```python
from build123d import *

# Parameters (mm, degrees)
F1_DEPTH = 101.6
F2_DEPTH = 12.7
F3_DEPTH = 57.15
F0_W     = 14.5453011187
F0_H     = 10.745606224
F4_DEPTH = 57.15
F6_R     = 25.4
F7_DEPTH = 12.7


# Not quite as in the source:
# - a feature names something its author has since deleted; it is built from what else it names


with BuildPart() as f1:
    # F0 (on Right) → F1 (new body, symmetric)
    with BuildSketch(Plane.YZ):
        Polygon((31.0628309338, 12.7), (-46.3495767937, 12.7), (-46.3495767937, -12.7), (46.3495767937, -12.7), (46.3495767937, 12.7), align=None)
    extrude(amount=F1_DEPTH, both=True)

    # F0 (on Right) → F2 (join, symmetric)
    with BuildSketch(Plane.YZ):
        Polygon((31.0628309338, 58.703106785), (-46.3495767937, 12.7), (31.0628309338, 12.7), align=None)
    extrude(amount=F2_DEPTH, both=True)

    # F0 (on Right) → F3 (join, symmetric)
    with BuildSketch(Plane.YZ):
        Polygon((31.0628309338, 58.703106785), (31.0628309338, 12.7), (46.3495767937, 12.7), (46.3495767937, 47.9575005611), (78.0453036841, 47.9575005611), (78.0453036841, 58.703106785), align=None)
    extrude(amount=F3_DEPTH, both=True)

    # F0 (on Right) → F4 (join, symmetric)
    with BuildSketch(Plane.YZ):
        with Locations((85.3179542435, 53.330303673)):
            Rectangle(F0_W, F0_H)
    extrude(amount=F4_DEPTH, both=True)

    # F0 (on Right) → F5 (revolve)
    with BuildSketch(Plane.YZ):
        Polygon((92.5906048029, 65.6709397763), (92.5906048029, 58.703106785), (92.5906048029, 47.9575005611), (92.5906048029, 36.5803426697), (107.1359059216, 36.5803426697), (107.1359059216, 65.6709397763), align=None)
    revolve(axis=Axis((0, 92.5906048029, 51.125641223), (0, 0, -1)))

    # F6 (on Top) → F7 (cut, symmetric)
    with BuildSketch(Plane.XY):
        with Locations((-63.5, 0)):
            Circle(F6_R)
        with Locations((63.5, 0)):
            Circle(F6_R)
    extrude(amount=F7_DEPTH, both=True, mode=Mode.SUBTRACT)


solid = f1.part
```
Check sheet for the modelled part. Datum: model origin and axes. Units: mm. A direction names the side the tool comes from. Round coordinates to 2 decimals unless told otherwise and drop trailing zeros. Order: outer loops, then holes, each group sorted by start corner. A loop starts at its lowest first (then second) coordinate and runs counter-clockwise, first axis right, second up. Notation, with made-up numbers: (-27.5, -10.5) - (5.5, -10.5) arc R13 cw to (5.5, 12.5) - close; hole circle Ø9 at (9.25, 45). An arc over 180 degrees is marked (long way). Answer as CSV lines item,"result". Start each with the question number.
1) Scan lines: probe 1 along Y at (x, z) = (-63, 4); probe 2 along Z at (x, y) = (-18, 82.5); probe 3 along X at (y, z) = (39, 47). Record each from-to range of solid material in increasing order.
2) Section check B-B (y = 6.5). Record the cut outline in (x, z), then the cut area to 3 significant figures.
3) Tool access check on faces 4 (the face through (36, 92.591, 53)), 5 (the face through (-36, 92.591, 53)), 6 (the face through (0, 93, 36.58)), 7 (the face through (35, 31.063, 36)). Record the directions out of +Z, -Z, +X, -X, +Y, -Y that give a thin tool (end or side, any length) a straight path to the whole face; none if there is none.
4) Section check C-C (z = 43). Record the cut outline in (x, y).
5) Depth check by flat-ended pin: pin 1 (14.5 mm diameter, centred on x = -1.5, y = 99.5, fed in from -Z); pin 2 (6 mm diameter, centred on x = -41, z = 43, fed in from +Y); pin 3 (5.5 mm diameter, centred on x = -33.5, z = 53.5, fed in from +Y). Enter the tip coordinate at first touch or a pass-through.
6) Draft check along Y on faces 1 (the face through (-57.15, 48, 51)), 2 (the face through (87.727, 7.629, 0.178)), 3 (the face through (1, -46.35, 0)). Enter one of: +Y half, -Y half, draft (parallel to the pull), parting line (faces both ways), or undercut.
7) Section check D-D (x = 0). Record the cut outline in (y, z), then the cut area to 3 significant figures.
8) Section check A-A (x = -63.5). Record the cut outline in (y, z), then the cut area to 3 significant figures.
Determined:
1,probe 1,"-46.35 to -25.4, 25.4 to 46.35"
1,probe 2,"47.96 to 58.7"
1,probe 3,"-57.15 to 57.15"
2,outline,"(-101.6, -12.7) - (-88.05, -12.7) - (-88.05, 12.7) - (-101.6, 12.7) - close; (-38.95, -12.7) - (38.95, -12.7) - (38.95, 12.7) - (12.7, 12.7) - (12.7, 44.11) - (-12.7, 44.11) - (-12.7, 12.7) - (-38.95, 12.7) - close; (88.05, -12.7) - (101.6, -12.7) - (101.6, 12.7) - (88.05, 12.7) - close"
2,area,"3,460 mm^2"
3,face 4,"+Z, -Z, +X, +Y"
3,face 5,"+Z, -Z, -X, +Y"
3,face 6,"-Z, +X, -X, +Y"
3,face 7,"+Z, +X, -Y"
4,outline,"(-57.15, 31.06) - (-12.7, 31.06) - (-12.7, 4.64) - (12.7, 4.64) - (12.7, 31.06) - (57.15, 31.06) - (57.15, 46.35) - (-57.15, 46.35) - close; circle Ø29.09 at (0, 92.59)"
5,pin 1,"z = 36.58"
5,pin 2,"y = 46.35"
5,pin 3,"y = 92.59"
6,face 1,"draft"
6,face 2,"undercut"
6,face 3,"-Y half"
7,outline,"(-46.35, -12.7) - (46.35, -12.7) - (46.35, 47.96) - (78.05, 47.96) - (78.05, 36.58) - (107.14, 36.58) - (107.14, 65.67) - (78.05, 65.67) - (78.05, 58.7) - (31.06, 58.7) - (-46.35, 12.7) - close"
7,area,"6,030 mm^2"
8,outline,"(-46.35, -12.7) - (-25.4, -12.7) - (-25.4, 12.7) - (-46.35, 12.7) - close; (25.4, -12.7) - (46.35, -12.7) - (46.35, 12.7) - (25.4, 12.7) - close"
8,area,"1,060 mm^2"
